The drawing under review shows one solid part. Ordinate dimensions are in mm from its lowest x, y, z. A direction names the side the tool comes from. Coordinates: 2 decimals unless noted, no trailing zeros. Write each loop counter-clockwise with the first axis right and the second up, starting at its lowest first coordinate (ties: lowest second). Pieces come first, ordered by that corner, then holes.
1) For P1, Ø2.5, axis at y = 33.5, z = 2, coming from the +X side; P2, Ø2.5, axis at y = 33.5, z = 2.5, coming from the -X side, all flat-tipped, find the tip position at first contact; note any pin that passes through.
2) Add section A-A, the plane x = 54. State the section outline as (y, z) points.
3) Mouldability with a two-part tool opening along X and no side actions: class the marked faces 3, 4, 5 and 6 as released by +X, released by -X, zero draft, split by the parting line, or undercut.
4) Add section D-D, the plane x = 38. State the section outline as (y, z) points, then the cut area to 3 significant figures.
5) For line 1 (Y direction, x = 38, z = 2.35); line 2 (Y direction, x = 5, z = 1.3); line 3 (Y direction, x = 71.5, z = 4.45), list the stretches that pass through material, from the lowest coordinate up.
6) Add section C-C, the plane z = 2.3. Give the number of separate pieces and of enclosed holes in the cut face, then the cut area to 3 significant figures.
7) Add section B-B, the plane y = 10. State the section outline as (x, z) points, then the cut area to 3 significant figures.
8) Machinability: for the marked faces 1 and 2, which of the approach directions +Z, -Z, +X, -X, +Y, -Y give a long, thin tool a straight path to every point of the face, cutting with its end or side? Answer none if there is none.
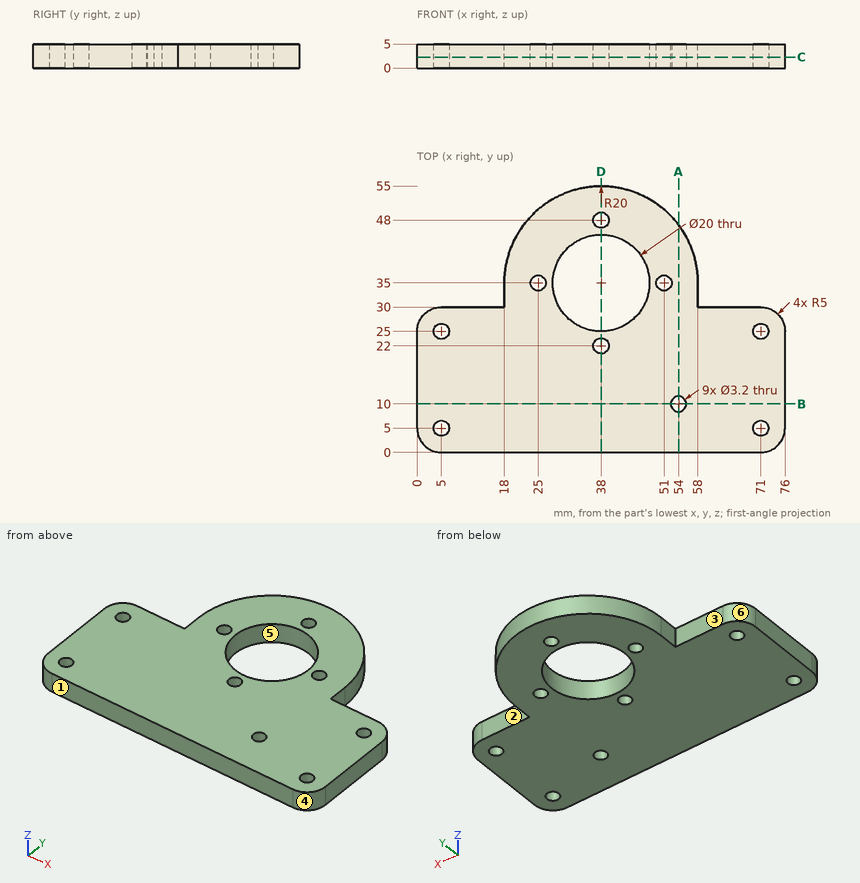
Geometry results:
1. P1: stops at x = 58
1. P2: stops at x = 18
2. outline: (0, 0) - (8.4, 0) - (8.4, 5) - (0, 5) - close; (11.6, 0) - (47, 0) - (47, 5) - (11.6, 5) - close
3. face 3: zero draft
3. face 4: released by +X
3. face 5: undercut
3. face 6: released by -X
4. outline: (0, 0) - (20.4, 0) - (20.4, 5) - (0, 5) - close; (23.6, 0) - (25, 0) - (25, 5) - (23.6, 5) - close; (45, 0) - (46.4, 0) - (46.4, 5) - (45, 5) - close; (49.6, 0) - (55, 0) - (55, 5) - (49.6, 5) - close
4. area: 143 mm2
5. line 1: y = 0 to 20.4, 23.6 to 25, 45 to 46.4, 49.6 to 55
5. line 2: y = 0 to 3.4, 6.6 to 23.4, 26.6 to 30
5. line 3: y = 0.03 to 3.48, 6.52 to 23.48, 26.52 to 29.97
6. separate pieces: 1
6. enclosed holes: 10
6. area: 2,700 mm2
7. outline: (0, 0) - (52.4, 0) - (52.4, 5) - (0, 5) - close; (55.6, 0) - (76, 0) - (76, 5) - (55.6, 5) - close
7. area: 364 mm2
8. face 1: +Z, -Z, +X, -X, -Y
8. face 2: +Z, -Z, +X, +Y
